Part model, mm, in its own coordinate system. A direction names the side the tool comes from. Give positions to 0.01 mm unless a question says otherwise; leave off trailing zeros. Order: outer loops, then holes, each group sorted by start corner. A loop starts at its lowest first (then second) coordinate and runs counter-clockwise, first axis right, second up. Notation, with made-up numbers: M 53.5,3 L 109.5,3 A19 ccw 109.5,10 Z; hole C 15.25,5 d3. An arc over 180 degrees is marked long. Return JSON: item names as keys, results as strings.
from build123d import *

# Parameters (mm, degrees)
SKETCH_1_W          = 88.8
SKETCH_1_H          = 103.8
EXTRUDE_1_DEPTH     = 1.5
SKETCH_2_W          = 85.5
SKETCH_2_H          = 100.5
SKETCH_2_W_2        = 82.5
SKETCH_2_H_2        = 97.5
EXTRUDE_2_DEPTH     = 3
EXTRUDE_3_DEPTH     = 6
SKETCH_6_W          = 10.5
SKETCH_6_H          = 6
SKETCH_6_W_2        = 15.5
SKETCH_6_W_3        = 10.4
CUT_EXTRUDE_2_DEPTH = 1.5
SKETCH_7_R          = 1.5
SKETCH_7_W          = 15.5
SKETCH_7_H          = 10
SKETCH_7_W_2        = 12
SKETCH_7_H_2        = 16
SKETCH_7_W_3        = 2.325623679
SKETCH_7_H_3        = 2
SKETCH_7_W_4        = 4.188972838
SKETCH_7_W_5        = 5
SKETCH_7_H_4        = 4
CUT_EXTRUDE_5_DEPTH = 10


with BuildPart() as part:
    # 草图1 → 凸台-拉伸1 (new body)
    with BuildSketch(Plane(origin=(0, 0, 0), x_dir=(1, 0, 0), z_dir=(0, 1, 0))):
        Rectangle(SKETCH_1_W, SKETCH_1_H)
    extrude(amount=EXTRUDE_1_DEPTH)

    # 草图2 → 凸台-拉伸2 (add)
    with BuildSketch(Plane(origin=(0, 1.5, 0), x_dir=(1, 0, 0), z_dir=(0, 1, 0))):
        Rectangle(SKETCH_2_W, SKETCH_2_H)
        Rectangle(SKETCH_2_W_2, SKETCH_2_H_2, mode=Mode.SUBTRACT)
    extrude(amount=EXTRUDE_2_DEPTH)

    # 草图3 → 凸台-拉伸3 (add)
    with BuildSketch(Plane.ZY.offset(42.75)):
        Polygon((5, 12.5), (-5, 12.5), (-5, 4.5), (-5, 1.5), (5, 1.5), (5, 4.5), align=None)
        Polygon((0, 11.964101615), (-3, 10.232050808), (-3, 6.767949192), (0, 5.035898385), (3, 6.767949192), (3, 10.232050808), align=None, mode=Mode.SUBTRACT)
    extrude(amount=-EXTRUDE_3_DEPTH)

    # 草图6 → 切除-拉伸2 (cut)
    with BuildSketch(Plane(origin=(0, 0, -50.25), x_dir=(-1, 0, 0), z_dir=(0, 0, -1))):
        with Locations((23.65, 4.5)):
            Rectangle(SKETCH_6_W, SKETCH_6_H)
        with Locations((-26.05, 4.5)):
            Rectangle(SKETCH_6_W_2, SKETCH_6_H)
        with Locations((-3.7, 4.5)):
            Rectangle(SKETCH_6_W_3, SKETCH_6_H)
    extrude(amount=-CUT_EXTRUDE_2_DEPTH, mode=Mode.SUBTRACT)

    # 草图7 → 切除-拉伸5 (cut)
    with BuildSketch(Plane(origin=(0, 0, 0), x_dir=(1, 0, 0), z_dir=(0, 1, 0))):
        with Locations((-38.75, 11)):
            Circle(SKETCH_7_R)
        with Locations((26.05, -45.25)):
            Rectangle(SKETCH_7_W, SKETCH_7_H)
        with Locations((4.6, -42.25)):
            Rectangle(SKETCH_7_W_2, SKETCH_7_H_2)
        with Locations((-24.4, -42.25)):
            Rectangle(SKETCH_7_W_2, SKETCH_7_H_2)
        with Locations((13.76281184, -41.25)):
            Rectangle(SKETCH_7_W_3, SKETCH_7_H_3)
        with Locations((-16.205513581, -39.25)):
            Rectangle(SKETCH_7_W_4, SKETCH_7_H_3)
        with Locations((-26, -5.25)):
            Rectangle(SKETCH_7_W_5, SKETCH_7_H_4)
    extrude(amount=CUT_EXTRUDE_5_DEPTH, mode=Mode.SUBTRACT)


solid = part.part
Q1. Band-saw the part on A-A (y = 8.75). Give the cut face in (x, z).
Established:
{"outline": "M -42.75,-5 L -36.75,-5 L -36.75,-3 L -42.75,-3 Z; M -42.75,3 L -36.75,3 L -36.75,5 L -42.75,5 Z"}
Q2. 3-axis set-ups, long thin cutter, end or side, ignore diameter. For faces 4 (the flat face through (-40, 7, -5)), 5 (the flat face through (42.75, 3, 1)), 6 (the flat face through (-40, 8, 3)), 7 (the flat face through (-1.4, 1, 44)), 8 (the flat face through (-10, 3, 50.25)): which of +Z, -Z, +X, -X, +Y, -Y reach the whole face in a straight line?
Established:
{"face 4": "+Y", "face 5": "+Z, -Z, +X, +Y", "face 6": "+X, -X", "face 7": "+Y, -Y", "face 8": "+Z, +X, -X, +Y"}
Q3. Band-saw the part on C-C (x = -38.75). Give the cut face in (y, z).
Established:
{"outline": "M 0,-51.9 L 1.5,-51.9 L 1.5,-50.25 L 4.5,-50.25 L 4.5,-48.75 L 1.5,-48.75 L 1.5,-12.5 L 0,-12.5 Z; M 0,-9.5 L 1.5,-9.5 L 1.5,-5 L 12.5,-5 L 12.5,5 L 1.5,5 L 1.5,48.75 L 4.5,48.75 L 4.5,50.25 L 1.5,50.25 L 1.5,51.9 L 0,51.9 Z; hole M 5.04,0 L 6.77,-3 L 10.23,-3 L 11.96,0 L 10.23,3 L 6.77,3 Z"}
Q4. Pin check, flat tips, straight feed: pin 1 (5 mm diameter, centred on y = 6.5, z = 24.5, fed in from +X); pin 2 (2.5 mm diameter, centred on x = 15, y = 3, fed in from -Z); pin 3 (5 mm diameter, centred on y = 8.5, z = -32.5, fed in from +X); pin 4 (3 mm diameter, centred on x = -39, y = 8, fed in from +Z). Stop position of each tip, or through.
Established:
{"pin 1": "stops at x = 42.75", "pin 2": "stops at z = -50.25", "pin 3": "passes through", "pin 4": "stops at z = 5"}
Q5. Two-plate mould, pull along Z, no slides. Class faces 1 (the flat face through (-37, 3, 50.25)), 2 (the flat face through (18.3, 1, 46)), 3 (the flat face through (-42.75, 4, 0)): +Z half, -Z half, draft (parallel to the pull), parting line (faces both ways), or undercut.
Established:
{"face 1": "+Z half", "face 2": "undercut", "face 3": "draft"}
Q6. Band-saw the part on D-D (z = -11). Give the cut face in (x, y), then the cut area to 3 significant figures.
Established:
{"outline": "M -44.4,0 L -40.25,0 L -40.25,1.5 L -41.25,1.5 L -41.25,4.5 L -42.75,4.5 L -42.75,1.5 L -44.4,1.5 Z; M -37.25,0 L 44.4,0 L 44.4,1.5 L 42.75,1.5 L 42.75,4.5 L 41.25,4.5 L 41.25,1.5 L -37.25,1.5 Z", "area": "138 mm²"}
Q7. Probe line 1 along Z through (x, y) = (-38.75, 0.75); line 2 along X through (y, z) = (4, -32); line 3 along X through (y, z) = (0.5, -11). List the from-to ranges inside material, lowest first.
Established:
{"line 1": "z = -51.9 to -12.5, -9.5 to 51.9", "line 2": "x = -42.75 to -41.25, 41.25 to 42.75", "line 3": "x = -44.4 to -40.25, -37.25 to 44.4"}
Q8. Band-saw the part on B-B (x = 24.5). Give the cut face in (y, z).
Established:
{"outline": "M 0,-51.9 L 1.5,-51.9 L 1.5,40.25 L 0,40.25 Z; M 0,50.25 L 1.5,50.25 L 1.5,51.9 L 0,51.9 Z"}
